The drawing under review shows one solid part. Ordinate dimensions are in mm from its lowest x, y, z. Give positions to 0.01 mm unless a question says otherwise; leave off trailing zeros. Write each loop counter-clockwise with the first axis right and the second up, starting at its lowest first coordinate (ties: lowest second). Pieces come first, ordered by that corner, then holes.
Q1. For line 1 (Y direction, x = 15, z = 1.25), list the stretches that pass through material, from the lowest coordinate up.
Q2. We need section A-A (y = 15). Write out the cut boundary in (x, z).
Q3. We need section B-B (x = 61). Write out the cut boundary in (y, z), then the cut area to 3 significant figures.
Q4. Insertion check: P1, Ø4, axis at x = 61, y = 97.5, coming from the +Z side; P2, Ø8.5, axis at x = 15, y = 97.5, coming from the -Z side. Each pin has a flat end and moves straight along its axis. Give the tip position at first contact, or say it passes through.
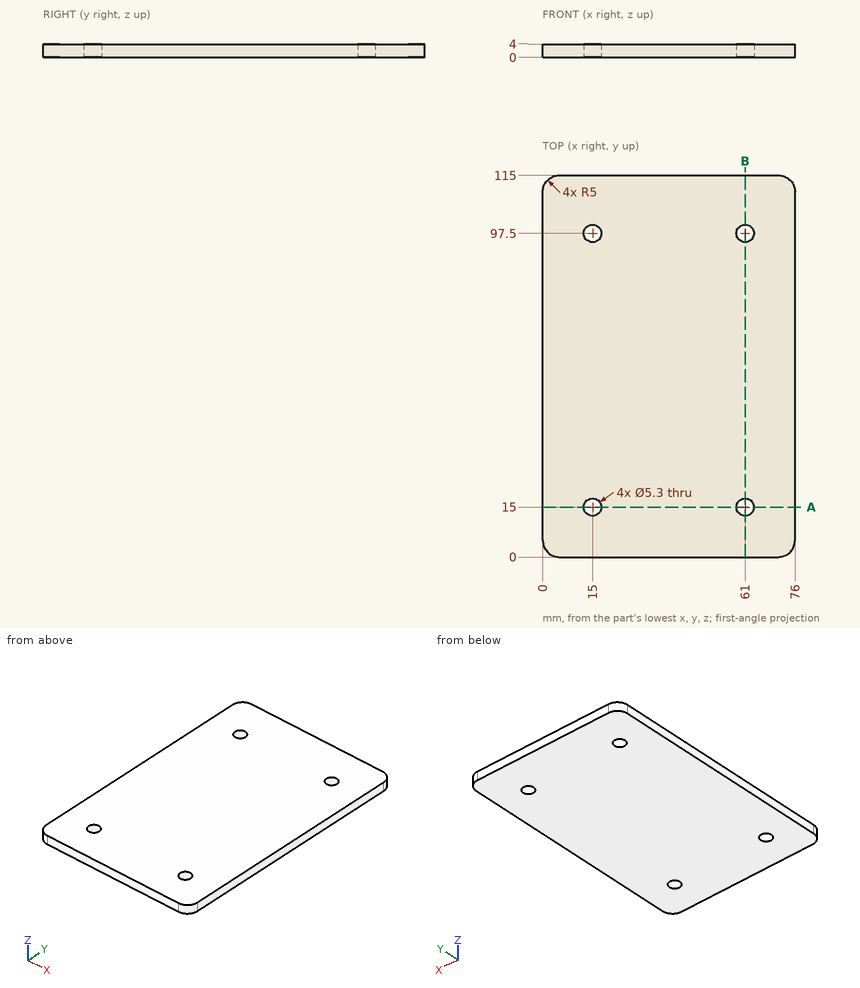
Computed:
1. line 1: y = 0 to 12.35, 17.65 to 94.85, 100.15 to 115
2. outline: (0, 0) - (12.35, 0) - (12.35, 4) - (0, 4) - close; (17.65, 0) - (58.35, 0) - (58.35, 4) - (17.65, 4) - close; (63.65, 0) - (76, 0) - (76, 4) - (63.65, 4) - close
3. outline: (0, 0) - (12.35, 0) - (12.35, 4) - (0, 4) - close; (17.65, 0) - (94.85, 0) - (94.85, 4) - (17.65, 4) - close; (100.15, 0) - (115, 0) - (115, 4) - (100.15, 4) - close
3. area: 418 mm2
4. P1: passes through
4. P2: stops at z = 0
